The figure shows three views and two pictorial views of one solid part (mm, origin at its lowest corner). Answer the questions. A direction names the side the tool comes from. Round coordinates to 2 decimals unless told otherwise and drop trailing zeros. Write each loop counter-clockwise with the first axis right and the second up, starting at its lowest first coordinate (ties: lowest second). Pieces come first, ordered by that corner, then holes.
Item 1: Find section D-D on z = 17.5. Give the vertices of the cut face in (x, y), then the cut area to 3 significant figures.
Item 2: A tool of negligible diameter and unlimited length cuts with its end or side. For the marked faces 1, 2 and 3, from which of +Z, -Z, +X, -X, +Y, -Y can it reach the whole face along a straight path? Write none if from no direction.
Item 3: For a pull along X with two mould halves and no side action, classify the marked faces 4 and 5 as +X half, -X half, draft (parallel to the pull), parting line (faces both ways), or undercut.
Item 4: Find section B-B on x = 18.5. Give the vertices of the cut face in (y, z), then the cut area to 3 significant figures.
Item 5: Find section A-A on z = 65.5. Give the vertices of the cut face in (x, y), then the cut area to 3 significant figures.
Item 6: Each of these flat-tipped pins is pushed along its axis until it touches: pin 1 (3.5 mm diameter, centred on x = 34, y = 18.5, fed in from +Z); pin 2 (0.9 mm diameter, centred on x = 11.5, y = 5.5, fed in from +Z); pin 3 (2 mm diameter, centred on y = 8.5, z = 61, fed in from -X). Where does it stop, or does it pass through?
Item 7: Find the intervals of material crossed by probe 1 along X at (y, z) = (18, 68) (1 decimal); probe 2 along Y at (x, z) = (10, 66) (1 decimal); probe 3 along Z at (x, y) = (9, 13), in increasing order.
Item 8: Find section C-C on y = 15.5. Give the vertices of the cut face in (x, z) (1 decimal), then the cut area to 3 significant figures.
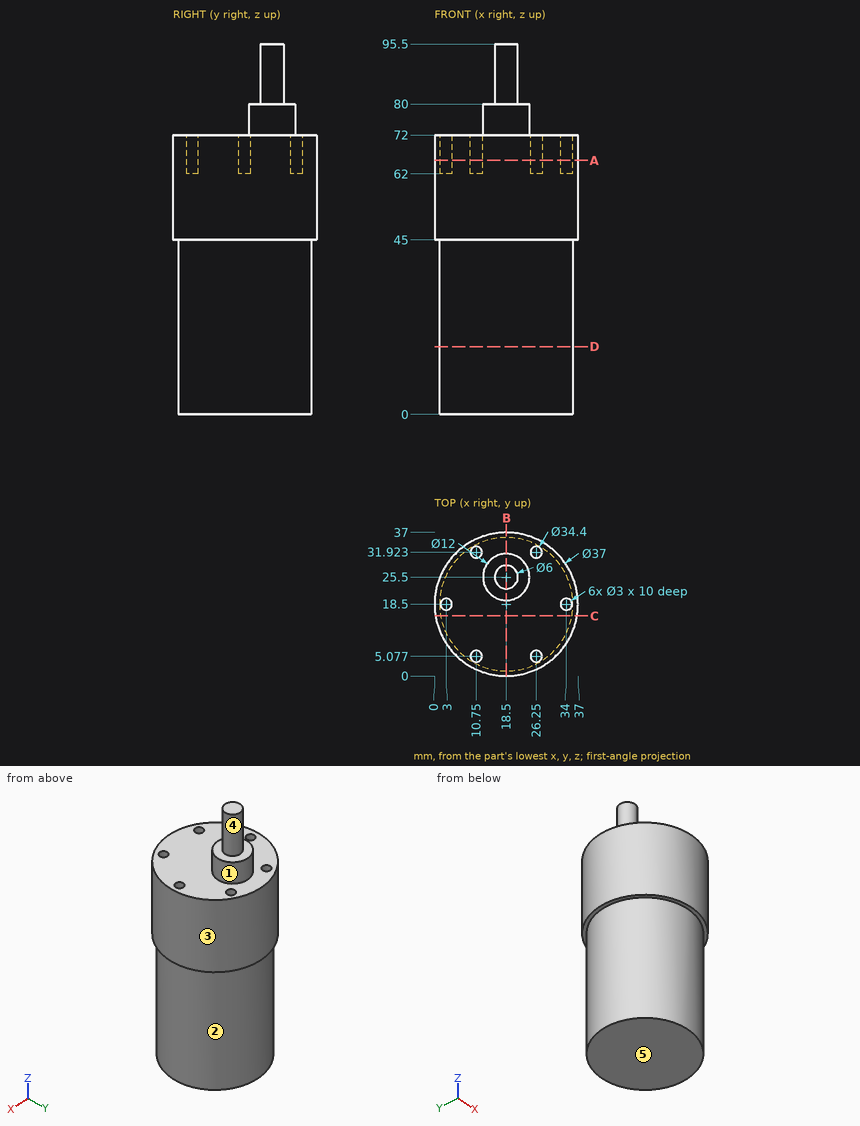
Check values:
1. outline: circle Ø34.4 at (18.5, 18.5)
1. area: 929 mm2
2. face 1: +Z
2. face 2: -Z
2. face 3: +Z, -Z
3. face 4: parting line
3. face 5: draft
4. outline: (0, 45) - (1.3, 45) - (1.3, 0) - (35.7, 0) - (35.7, 45) - (37, 45) - (37, 72) - (31.5, 72) - (31.5, 80) - (28.5, 80) - (28.5, 95.5) - (22.5, 95.5) - (22.5, 80) - (19.5, 80) - (19.5, 72) - (0, 72) - close
4. area: 2,740 mm2
5. outline: circle Ø37 at (18.5, 18.5); hole circle Ø3 at (3, 18.5); hole circle Ø3 at (10.75, 5.08); hole circle Ø3 at (10.75, 31.92); hole circle Ø3 at (26.25, 5.08); hole circle Ø3 at (26.25, 31.92); hole circle Ø3 at (34, 18.5)
5. area: 1,030 mm2
6. pin 1: stops at z = 72
6. pin 2: stops at z = 62
6. pin 3: stops at x = 2.34
7. probe 1: x = 0 to 1.6, 4.4 to 32.6, 35.4 to 37
7. probe 2: y = 2.1 to 3.8, 6.4 to 30.6, 33.2 to 34.9
7. probe 3: z = 0 to 72
8. outline: (0.2, 45) - (1.6, 45) - (1.6, 0) - (35.4, 0) - (35.4, 45) - (36.8, 45) - (36.8, 72) - (0.2, 72) - close
8. area: 2,510 mm2
